For this review, take the finished solid that the model builds, in its own axes (mm). A direction names the side the tool comes from. Coordinates: 2 decimals unless noted, no trailing zeros. Write each loop counter-clockwise with the first axis right and the second up, starting at its lowest first coordinate (ties: lowest second). Pieces come first, ordered by that corner, then holes.
```python
from build123d import *

# Parameters (mm, degrees)
SKETCH1_R              = 15
SKETCH1_R_2            = 10
BOSS_EXTRUDE1_DEPTH    = 55
M8_TAPPED_HOLE1_REACH  = 66.42
M8_TAPPED_HOLE1_BORE_R = 3.4
CHAMFER1_SIZE          = 1


with BuildPart() as part:
    # Sketch1 → Boss-Extrude1 (new body)
    with BuildSketch(Plane(origin=(0, 0, 0), x_dir=(1, 0, 0), z_dir=(0, 1, 0))):
        with Locations(Location((0, 0, 0), (0, 0, 270))):
            Circle(SKETCH1_R)
        with Locations(Location((0, 0, 0), (0, 0, 270))):
            Circle(SKETCH1_R_2, mode=Mode.SUBTRACT)
    extrude(amount=BOSS_EXTRUDE1_DEPTH)

    # M8 Tapped Hole1 bore → M8 Tapped Hole1 (cut, up to next)
    with BuildSketch(Plane.XY.offset(15), mode=Mode.PRIVATE) as m8_tapped_hole1_sk1:
        with Locations((0, 47)):
            Circle(M8_TAPPED_HOLE1_BORE_R)
    m8_tapped_hole1_tool1 = extrude(m8_tapped_hole1_sk1.sketch, amount=-M8_TAPPED_HOLE1_REACH, mode=Mode.PRIVATE) & part.part
    # M8 Tapped Hole1 bore → M8 Tapped Hole1 (cut, up to next)
    with BuildSketch(Plane.XY.offset(15), mode=Mode.PRIVATE) as m8_tapped_hole1_sk2:
        with Locations((0, 20)):
            Circle(M8_TAPPED_HOLE1_BORE_R)
    m8_tapped_hole1_tool2 = extrude(m8_tapped_hole1_sk2.sketch, amount=-M8_TAPPED_HOLE1_REACH, mode=Mode.PRIVATE) & part.part
    add(m8_tapped_hole1_tool1.solids().sort_by_distance((0, 47, 15))[0], mode=Mode.SUBTRACT)
    add(m8_tapped_hole1_tool2.solids().sort_by_distance((0, 20, 15))[0], mode=Mode.SUBTRACT)

    # Chamfer1
    chamfer1_edges = [part.edges().sort_by_distance(p)[0] for p in [
        (0, 55, -15),
    ]]
    chamfer(chamfer1_edges, length=CHAMFER1_SIZE)


solid = part.part
```
Q1. Add section B-B (z = 0). State the section outline as (x, y) points.
Ans:
outline: (-15, 0) - (-10, 0) - (-10, 55) - (-14, 55) - (-15, 54) - close; (10, 0) - (15, 0) - (15, 54) - (14, 55) - (10, 55) - close
Q2. Add section C-C (y = 12). State the section outline as (x, z) points.
Ans:
outline: circle Ø30 at (0, 0); hole circle Ø20 at (0, 0)
Q3. Add section A-A (x = 0). State the section outline as (y, z) points.
Ans:
outline: (0, -15) - (54, -15) - (55, -14) - (55, -10) - (0, -10) - close; (0, 10) - (16.6, 10) - (16.6, 15) - (0, 15) - close; (23.4, 10) - (43.6, 10) - (43.6, 15) - (23.4, 15) - close; (50.4, 10) - (55, 10) - (55, 14) - (54, 15) - (50.4, 15) - close
Q4. Clearance check with flat-ended pins moving along their axes: pin 1 Ø6 at (x, y) = (5, 34.5) entering from -Z; pin 2 Ø10 at (x, y) = (-5.5, 26) entering from -Z; pin 3 Ø6 at (y, z) = (34, 10) entering from +X. State where each tip first meets the part, or that it passes through.
Ans:
pin 1: stops at z = -14.87
pin 2: stops at z = -14.99
pin 3: stops at x = 13.27
Q5. Add section D-D (y = 22.5). State the section outline as (x, z) points, then the cut area to 3 significant figures.
Ans:
outline: (-2.3, 9.73) - (-2.3, 14.82) arc R15 ccw (long way) to (2.3, 14.82) - (2.3, 9.73) arc R10 cw (long way) to start
area: 370 mm2
Q6. For probe 1 along Y at (x, z) = (0, 12); probe 2 along X at (y, z) = (15, 0); probe 3 along Y at (x, z) = (-2, 10.5), list the stretches that pass through material, from the lowest coordinate up.
Ans:
probe 1: y = 0 to 16.6, 23.4 to 43.6, 50.4 to 55
probe 2: x = -15 to -10, 10 to 15
probe 3: y = 0 to 17.25, 22.75 to 44.25, 49.75 to 55
Q7. Tool access review of faces 1 (the cylindrical face through (-3.4, 20.1, 12.2)), 2 (the flat face through (10, 55, -3)): name each direction out of +Z, -Z, +X, -X, +Y, -Y from which nothing blocks a thin tool from reaching the whole face with its end or side.
Ans:
face 1: +Z
face 2: +Z, -Z, +X, -X, +Y
Q8. Draft analysis for pull direction Z (two halves, no side actions). For faces 3 (the cylindrical face through (-6, 27, -8)), 4 (the cylindrical face through (0.66, 26.622, -14.985)), 5 (the cylindrical face through (-3.4, 47.1, 12.2)), state which applies: +Z half, -Z half, draft (parallel to the pull), parting line (faces both ways), or undercut.
Ans:
face 3: undercut
face 4: parting line
face 5: draft
